Part model, mm, in its own coordinate system. A direction names the side the tool comes from. Round coordinates to 2 decimals unless told otherwise and drop trailing zeros. Loops run counter-clockwise (first coordinate to the right, second up) from the corner with the lowest first, then second, coordinate; pieces in that order, holes last.
(1) Cut at A-A on y = -18. List the corners of the cut face in (x, z), then the cut area to 3 significant figures.
(2) Cut at D-D on x = -17. List the corners of the cut face in (y, z), then the cut area to 3 significant figures.
(3) Probe probe 1 along X at (y, z) = (17.5, 4.55); probe 2 along Z at (x, y) = (-19.5, -28); probe 3 along Y at (x, z) = (16.5, 4.6). List the from-to ranges inside material, lowest first.
(4) Flat gauge pins, fed straight in: pin 1 (2 mm diameter, centred on x = -2, z = 1, fed in from -Y); pin 2 (1.6 mm diameter, centred on y = -8, z = 1.5, fed in from -X); pin 3 (1.5 mm diameter, centred on y = 15.5, z = 1.5, fed in from +X). Where does each tip first touch, or does it go through?
(5) Tool access for faces 4 (the face through (3, -26.622, 3)), 5 (the face through (1.39, 40.36, 1.42)): list every direction of +Z, -Z, +X, -X, +Y, -Y with a clear straight run to the whole face (end or side of a thin tool).
(6) Cut at C-C on y = -30. List the corners of the cut face in (x, z), then the cut area to 3 significant figures.
(7) Cut at B-B on x = 15.5. List the corners of the cut face in (y, z), then the cut area to 3 significant figures.
(8) Mould opens along X. For faces 1 (the face through (20, 0, 0)), 2 (the face through (29.35, 41.04, 3.89)), 3 (the face through (-26.5, -0.1, 1.4)) say: +X half, -X half, draft (parallel to the pull), parting line (faces both ways), or undercut.
from build123d import *

# Parameters (mm, degrees)
F0_W        = 69.0733827651
F0_H        = 94.4002903998
F0_R        = 1.9306579711
F0_W_2      = 31.083021313
F0_H_2      = 51.8050361425
F0_R_2      = 2.0350948247
F1_DEPTH    = 5.334
F2_T1_DEPTH = 136.319889095
F2_T3_DEPTH = 161.6467967298


# Not quite as in the source:
# - a fillet or chamfer that OpenCascade refuses, or shapes differently, is made with other operations: its cross-section is extruded or revolved along the edge and cut away or added


with BuildPart() as f1:
    # F0 (on Top) → F1 (new body)
    with BuildSketch(Plane.XY):
        with Locations((1.8707383424, -0.7195156068)):
            Rectangle(F0_W, F0_H)
        with Locations((-26.0464213789, 42.1635434031)):
            Circle(F0_R, mode=Mode.SUBTRACT)
        with Locations((3.021961078, -0.7195146754)):
            Rectangle(F0_W_2, F0_H_2, mode=Mode.SUBTRACT)
        with Locations((29.7878980637, 43.0269613862)):
            Circle(F0_R_2, mode=Mode.SUBTRACT)
    extrude(amount=F1_DEPTH)

    # F2: fillet of radius 19.622727835 on 4 edges, made by hand

    # F2_s2 → F2_t1 (cut)
    with BuildSketch(Plane.YZ.offset(-66.2892062051)):
        with BuildLine():
            ThreePointArc((46.4806295931, 5.334), (40.2655397656, 1.3821787054), (33.0313283271, 0))
            Line((33.0313283271, 0), (46.4806295931, 0))
            Line((46.4806295931, 0), (46.4806295931, 5.334))
        make_face()
        with BuildLine():
            ThreePointArc((-47.9196608067, 5.334), (-41.7045709791, 1.3821787054), (-34.4703595407, 0))
            Line((-34.4703595407, 0), (-47.9196608067, 0))
            Line((-47.9196608067, 0), (-47.9196608067, 5.334))
        make_face()
    extrude(amount=F2_T1_DEPTH, mode=Mode.SUBTRACT)

    # F2_s4 → F2_t3 (cut)
    with BuildSketch(Plane.XZ.offset(-80.1038827581)):
        with BuildLine():
            ThreePointArc((36.4074297249, 5.334), (30.1923398974, 1.3821787054), (22.9581284589, 0))
            Line((22.9581284589, 0), (36.4074297249, 0))
            Line((36.4074297249, 0), (36.4074297249, 5.334))
        make_face()
        with BuildLine():
            ThreePointArc((-32.6659530401, 5.334), (-26.4508632126, 1.3821787054), (-19.2166517741, 0))
            Line((-19.2166517741, 0), (-32.6659530401, 0))
            Line((-32.6659530401, 0), (-32.6659530401, 5.334))
        make_face()
    extrude(amount=F2_T3_DEPTH, mode=Mode.SUBTRACT)


solid = f1.part
Final values:
1. outline: (-32.67, 5.33) arc R19.62 ccw to (-19.22, 0) - (-12.52, 0) - (-12.52, 5.33) - close; (18.56, 0) - (22.96, 0) arc R19.62 ccw to (36.41, 5.33) - (18.56, 5.33) - close
1. area: 158 mm2
2. outline: (-47.92, 5.33) arc R19.62 ccw to (-34.47, 0) - (33.03, 0) arc R19.62 ccw to (46.48, 5.33) - close
2. area: 459 mm2
3. probe 1: x = -31.78 to -12.52, 18.56 to 35.52
3. probe 2: z = 0 to 5.33
3. probe 3: y = -47.09 to -26.62, 25.18 to 45.66
4. pin 1: stops at y = -43.1
4. pin 2: stops at x = -28.43
4. pin 3: stops at x = 32.08
5. face 4: +Z, -Z
5. face 5: -Z, +X, -X, +Y
6. outline: (-32.67, 5.33) arc R19.62 ccw to (-19.22, 0) - (22.96, 0) arc R19.62 ccw to (36.41, 5.33) - close
6. area: 324 mm2
7. outline: (-47.92, 5.33) arc R19.62 ccw to (-34.47, 0) - (-26.62, 0) - (-26.62, 5.33) - close; (25.18, 0) - (33.03, 0) arc R19.62 ccw to (46.48, 5.33) - (25.18, 5.33) - close
7. area: 182 mm2
8. face 1: draft
8. face 2: undercut
8. face 3: -X half
